For this review, use the dimensioned drawing (mm, ordinates from the lowest corner) and the shaded views. A direction names the side the tool comes from. Coordinates: 2 decimals unless noted, no trailing zeros. Order: outer loops, then holes, each group sorted by start corner. A loop starts at its lowest first (then second) coordinate and runs counter-clockwise, first axis right, second up. Notation, with made-up numbers: (-6.5, 8) -> (41.5, 8) arc R29 ccw to (41.5, 45) -> close; hole circle Ø7 at (-18.75, -13). An arc over 180 degrees is marked (long way). Use one line per item in the form item = value. Start each with the question number.
(1) Take a section at D-D (z = 124.5). State the section outline as (x, y) points, then the cut area to 3 significant figures.
(2) For the marked faces 1, 2 and 3, list the 3-axis set-ups (+Z, -Z, +X, -X, +Y, -Y) from which the entire face can be reached by the end or side of a thin tool; tool diameter is ignored.
(3) Insertion check: pin 1 Ø3 at (x, z) = (87, 42.5) entering from -Y. The pin has a flat end and moves straight along its axis. Give the tip position at first contact, or say it passes through.
(4) Take a section at A-A (z = 63.5). State the section outline as (x, y) points.
(5) Mouldability with a two-part tool opening along X and no side actions: class the marked faces 4, 5, 6 and 7 as +X half, -X half, draft (parallel to the pull), parting line (faces both ways), or undercut.
(6) Wall thickness on line 1 along Z through (x, y) = (76.5, 29.5) (1 decimal); line 2 along X through (y, z) = (47, 125.5); line 3 along X through (y, z) = (56, 108.5): over which ranges is each line inside the solid? List them lowest first.
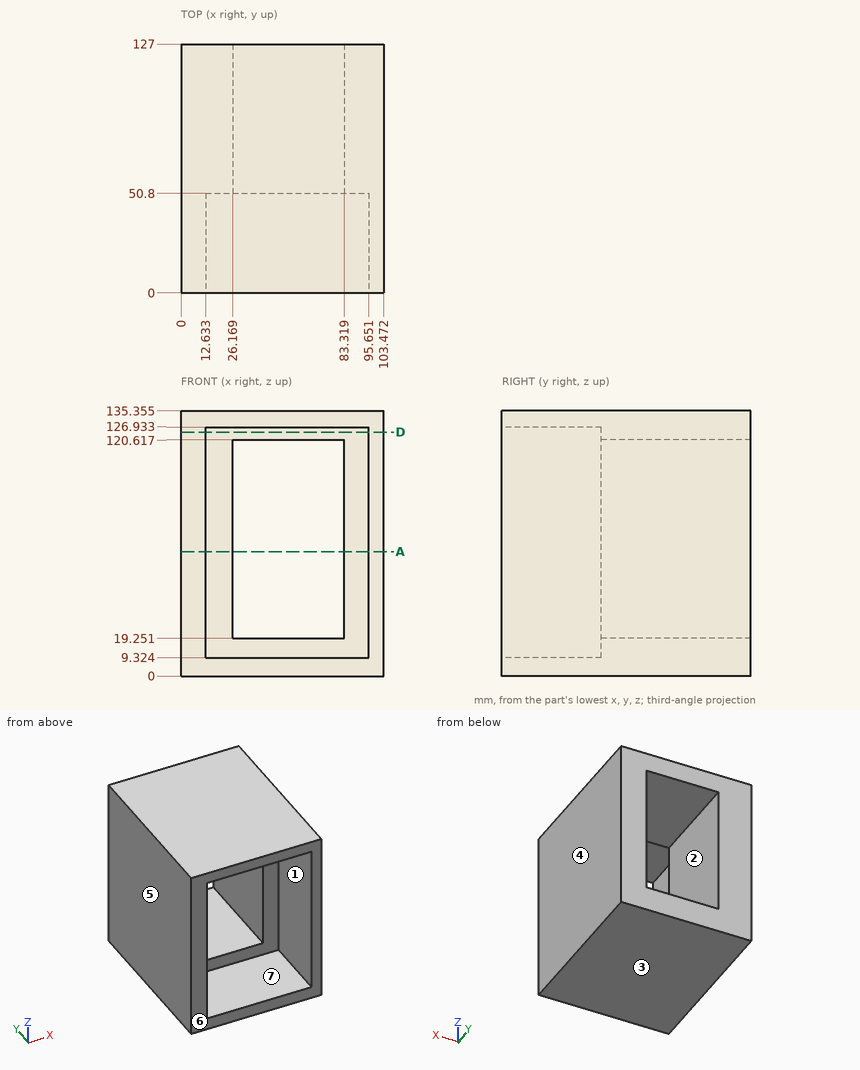
Findings:
q1.outline = (0, 0) -> (12.63, 0) -> (12.63, 50.8) -> (95.65, 50.8) -> (95.65, 0) -> (103.47, 0) -> (103.47, 127) -> (0, 127) -> close
q1.area = 8,920 mm²
q2.face_1 = -Y
q2.face_2 = +Y, -Y
q2.face_3 = -Z, +X, -X, +Y, -Y
q3.pin_1 = 50.8
q4.outline = (0, 0) -> (12.63, 0) -> (12.63, 50.8) -> (26.17, 50.8) -> (26.17, 127) -> (0, 127) -> close; (83.32, 50.8) -> (95.65, 50.8) -> (95.65, 0) -> (103.47, 0) -> (103.47, 127) -> (83.32, 127) -> close
q5.face_4 = +X half
q5.face_5 = -X half
q5.face_6 = draft
q5.face_7 = undercut
q6.line_1 = 0 to 9.3, 126.9 to 135.4
q6.line_2 = 0 to 12.63, 95.65 to 103.47
q6.line_3 = 0 to 26.17, 83.32 to 103.47
